Geometry: see drawing. Coordinates: mm, zero at the bounding-box minimum. A direction names the side the tool comes from. Coordinates: 2 decimals unless noted, no trailing zeros. Order: outer loops, then holes, each group sorted by start corner. A loop starts at its lowest first (then second) coordinate and runs counter-clockwise, first axis right, second up. Notation, with made-up numbers: (-28, 17) -> (7, 17) arc R20 cw to (7, 46) -> close; hole circle Ø5 at (42, -1.5). An arc over 180 degrees is marked (long way). Use one line per item in the form item = value.
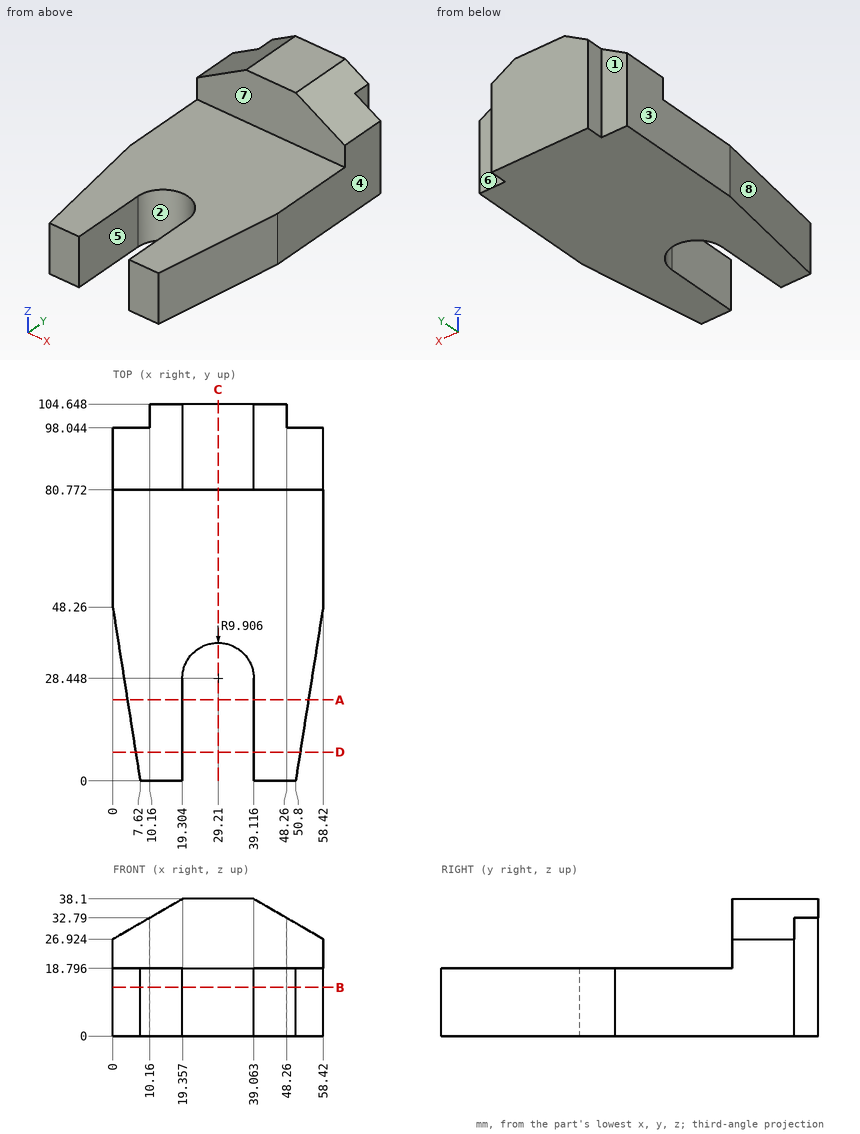
1) Section B-B, the plane z = 13.5. Output: boundary loops of the cut face in (x, y).
Results found:
outline = (0, 48.26) -> (7.62, 0) -> (19.3, 0) -> (19.3, 28.45) arc R9.91 cw to (39.12, 28.45) -> (39.12, 0) -> (50.8, 0) -> (58.42, 48.26) -> (58.42, 98.04) -> (48.26, 98.04) -> (48.26, 104.65) -> (10.16, 104.65) -> (10.16, 98.04) -> (0, 98.04) -> close
2) Material intervals for probe 1 along Y at (x, z) = (27.5, 26.5); probe 2 along Z at (x, y) = (39, 67); probe 3 along X at (y, z) = (22, 18) (1 decimal), sorted ascending. Write a range as from..to.
Results found:
probe_1 = 80.77..104.65
probe_2 = 0..18.8
probe_3 = 4.1..19.3, 39.1..54.3
3) Section C-C, the plane x = 29.21. Output: boundary loops of the cut face in (y, z).
Results found:
outline = (38.35, 0) -> (104.65, 0) -> (104.65, 38.1) -> (80.77, 38.1) -> (80.77, 18.8) -> (38.35, 18.8) -> close
4) Access query for the marked faces 5, 6, 7 and 8. Directions: +Z, -Z, +X, -X, +Y, -Y. A direction counts if a zero-diameter tool reaches every point of the face in a straight line with its end or side. Return the directions, or none.
Results found:
face_5 = +Z, -Z, -Y
face_6 = +Z, -Z, +X, +Y
face_7 = +Z, +X, -X, -Y
face_8 = +Z, -Z, -X, -Y
5) Pull-direction query (X, two-part tool) for the marked faces 1, 2, 3 and 4; classes: released by +X, released by -X, zero draft, split by the parting line, or undercut.
Results found:
face_1 = zero draft
face_2 = undercut
face_3 = released by -X
face_4 = released by +X
6) Section A-A, the plane y = 22.5. Output: boundary loops of the cut face in (x, z), and give its area (3 significant figures).
Results found:
outline = (4.07, 0) -> (19.3, 0) -> (19.3, 18.8) -> (4.07, 18.8) -> close; (39.12, 0) -> (54.35, 0) -> (54.35, 18.8) -> (39.12, 18.8) -> close
area = 573 mm2
7) Section D-D, the plane y = 8. Output: boundary loops of the cut face in (x, z), and give its area (3 significant figures).
Results found:
outline = (6.36, 0) -> (19.3, 0) -> (19.3, 18.8) -> (6.36, 18.8) -> close; (39.12, 0) -> (52.06, 0) -> (52.06, 18.8) -> (39.12, 18.8) -> close
area = 487 mm2
8) Contact query for flat-ended pins moving along their axis: P1, Ø3, axis at x = 55, z = 20.5, coming from the +Y side; P2, Ø3.5, axis at y = 103, z = 17.5, coming from the -X side; P3, Ø5.5, axis at y = 21.5, z = 13, coming from the -X side. Output: stop coordinate, or through.
Results found:
P1 = 98.04
P2 = 10.16
P3 = 3.79
